```python
from build123d import *

# Parameters (mm, degrees)
BOSS_EXTRU_1_DEPTH = 5
CONG_1_R           = 5


with BuildPart() as part:
    # Esquisse1 → Boss.-Extru.1 (new body)
    with BuildSketch(Plane.XY):
        with BuildLine():
            Line((-79.883099041, 98.930477667), (-79.883099041, -51.069522333))
            Line((-79.883099041, -51.069522333), (-20.434042124, -51.069522333))
            Line((-20.434042124, -51.069522333), (-20.434042124, -45.101662771))
            Line((-20.434042124, -45.101662771), (-21.634042124, -45.101662771))
            Line((-21.634042124, -45.101662771), (-21.634042124, -42.681662771))
            Line((-21.634042124, -42.681662771), (-20.434042124, -42.681662771))
            Line((-20.434042124, -42.681662771), (-20.434042124, -36.069522333))
            Line((-20.434042124, -36.069522333), (-17.234042124, -36.069522333))
            Line((-17.234042124, -36.069522333), (-17.234042124, -42.681662771))
            Line((-17.234042124, -42.681662771), (-16.034042124, -42.681662771))
            Line((-16.034042124, -42.681662771), (-16.034042124, -45.101662771))
            Line((-16.034042124, -45.101662771), (-17.234042124, -45.101662771))
            Line((-17.234042124, -45.101662771), (-17.234042124, -51.069522333))
            Line((-17.234042124, -51.069522333), (3.640375371, -51.069522333))
            Line((3.640375371, -51.069522333), (3.640375371, -41.637138386))
            ThreePointArc((3.640375371, -41.637138386), (14.83816479, -30.439348967), (26.035954209, -41.637138386))
            Line((26.035954209, -41.637138386), (26.035954209, -51.069522333))
            Line((26.035954209, -51.069522333), (49.565957876, -51.069522333))
            Line((49.565957876, -51.069522333), (49.565957876, -45.101662771))
            Line((49.565957876, -45.101662771), (48.365957876, -45.101662771))
            Line((48.365957876, -45.101662771), (48.365957876, -42.681662771))
            Line((48.365957876, -42.681662771), (49.565957876, -42.681662771))
            Line((49.565957876, -42.681662771), (49.565957876, -36.069522333))
            Line((49.565957876, -36.069522333), (52.765957876, -36.069522333))
            Line((52.765957876, -36.069522333), (52.765957876, -42.681662771))
            Line((52.765957876, -42.681662771), (53.965957876, -42.681662771))
            Line((53.965957876, -42.681662771), (53.965957876, -45.101662771))
            Line((53.965957876, -45.101662771), (52.765957876, -45.101662771))
            Line((52.765957876, -45.101662771), (52.765957876, -51.069522333))
            Line((52.765957876, -51.069522333), (70.116900959, -51.069522333))
            Line((70.116900959, -51.069522333), (70.116900959, -43.569522333))
            Line((70.116900959, -43.569522333), (70.116900959, 71.449147664))
            Line((70.116900959, 71.449147664), (22.19472603, 81.384794059))
            Line((22.19472603, 81.384794059), (-48.758847586, -19.947410672))
            Line((-48.758847586, -19.947410672), (-64.883099041, -19.947410672))
            Line((-64.883099041, -19.947410672), (-64.883099041, 98.930477667))
            Line((-64.883099041, 98.930477667), (-79.883099041, 98.930477667))
        make_face()
    extrude(amount=BOSS_EXTRU_1_DEPTH)

    # Congé1
    cong_1_edges = [part.edges().sort_by_distance(p)[0] for p in [
        (-64.883099041, -19.947410672, 2.5),
        (-48.758847586, -19.947410672, 2.5),
    ]]
    fillet(cong_1_edges, radius=CONG_1_R)


solid = part.part
```
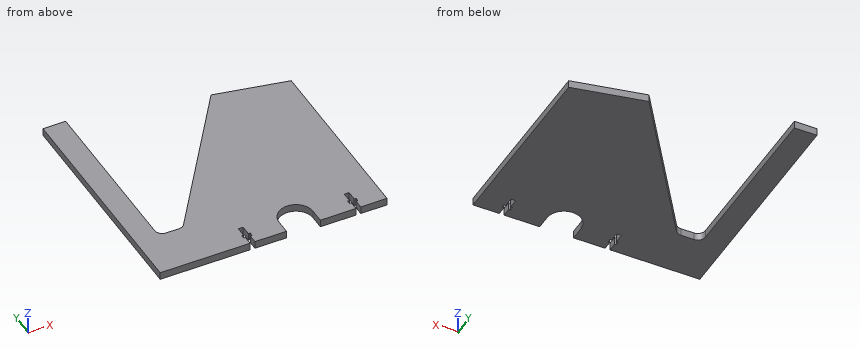
Work out the finished part from the listing and answer in its coordinate system (mm). Round coordinates to 2 decimals unless told otherwise and drop trailing zeros. Write each loop counter-clockwise with the first axis right and the second up, starting at its lowest first coordinate (ties: lowest second). Pieces come first, ordered by that corner, then holes.
1) Flat-ended cylindrical pins translate along their axes: P1, Ø0.6, axis at x = -16.5, z = 3, coming from the +Y side; P2, Ø0.6, axis at x = 49.5, z = 1.5, coming from the +Y side; P3, Ø1, axis at x = 53.5, z = 2.5, coming from the +Y side. Find the tip coordinate at first contact, or state that the pin passes through.
2) A cutting plane is placed at A-A on y = 67. Determine the outline of the cut face in (x, z).
3) A cutting plane is placed at D-D on x = -45. Determine the outline of the cut face in (y, z), and give its area (3 significant figures).
4) A cutting plane is placed at B-B on y = 37.5. Determine the outline of the cut face in (x, z), and give its area (3 significant figures).
5) Consider probe 1 along Y at (x, z) = (-52, 3.2); probe 2 along X at (y, z) = (4.5, 1.35); probe 3 along X at (y, z) = (6, 3.35). Determine where each line is inside the solid, lowest interval first.
6) A cutting plane is placed at C-C on y = 83.5. Determine the outline of the cut face in (x, z), and give its area (3 significant figures).
Entries:
1. P1: stops at y = 26.55
1. P2: stops at y = 75.79
1. P3: stops at y = 75
2. outline: (-79.88, 0) - (-64.88, 0) - (-64.88, 5) - (-79.88, 5) - close; (12.12, 0) - (70.12, 0) - (70.12, 5) - (12.12, 5) - close
3. outline: (-51.07, 0) - (-14.58, 0) - (-14.58, 5) - (-51.07, 5) - close
3. area: 182 mm2
4. outline: (-79.88, 0) - (-64.88, 0) - (-64.88, 5) - (-79.88, 5) - close; (-8.53, 0) - (70.12, 0) - (70.12, 5) - (-8.53, 5) - close
4. area: 468 mm2
5. probe 1: y = -51.07 to -19.95
5. probe 2: x = -79.88 to -64.88, -31.64 to 70.12
5. probe 3: x = -79.88 to -64.88, -30.59 to 70.12
6. outline: (-79.88, 0) - (-64.88, 0) - (-64.88, 5) - (-79.88, 5) - close
6. area: 75.0 mm2
